Study the drawing (mm; zero at the part's minimum x, y, z) and answer. A direction names the side the tool comes from. Coordinates: 2 decimals unless noted, no trailing zeros. Order: outer loops, then holes, each group sorted by start corner. A loop starts at its lowest first (then second) coordinate and runs counter-clockwise, first axis right, second up. Notation, with made-up numbers: (43, 39) -> (71, 39) arc R12 cw to (71, 49) -> close; hole circle Ø7 at (1, 64). An arc over 180 degrees is marked (long way). Put each result on its own line as item: value. Start each with the question number.
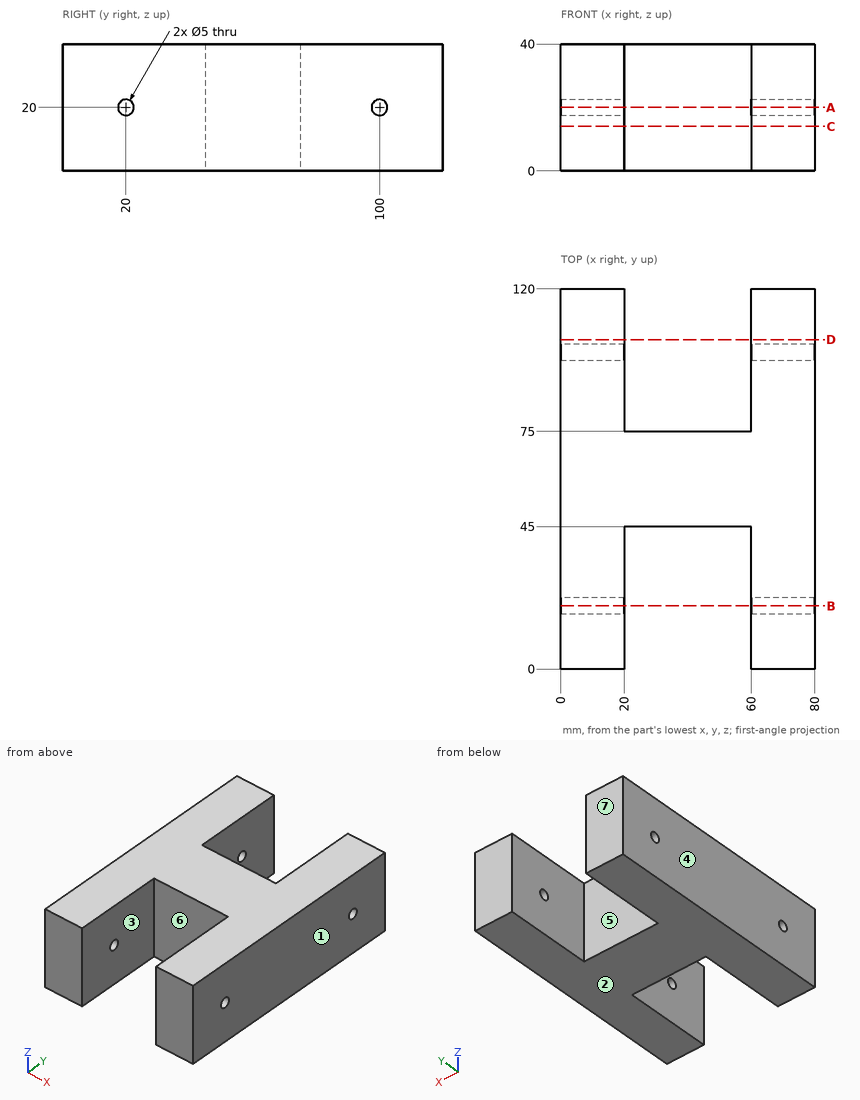
(1) For a pull along X with two mould halves and no side action, classify the marked faces 1, 2, 3 and 4 as released by +X, released by -X, zero draft, split by the parting line, or undercut.
(2) The part is cut by section C-C on z = 14. Determine the outline of the cut face in (x, y), plus the area to 3 significant figures.
(3) A tool of negligible diameter and unlimited length cuts with its end or side. For the marked faces 5, 6 and 7, from which of +Z, -Z, +X, -X, +Y, -Y can it reach the whole face along a straight path? Write none if from no direction.
(4) Find the intervals of material crossed by L1, parallel to Z at x = 70, y = 100; L2, parallel to X at y = 5, z = 8.5; L3, parallel to Y at x = 6, z = 22, in increasing order.
(5) Each of these flat-tipped pins is pushed along its axis until it touches: P1, Ø20, axis at x = 35, z = 20, coming from the +Y side; P2, Ø12, axis at x = 35.5, z = 21.5, coming from the -Y side. Where does it stop, or does it pass through?
(6) The part is cut by section B-B on y = 20. Determine the outline of the cut face in (x, z).
(7) The part is cut by section A-A on z = 20. Determine the outline of the cut face in (x, y).
(8) The part is cut by section D-D on y = 104. Determine the outline of the cut face in (x, z).
Worked out:
1. face 1: released by +X
1. face 2: zero draft
1. face 3: undercut
1. face 4: released by -X
2. outline: (0, 0) -> (20, 0) -> (20, 45) -> (60, 45) -> (60, 0) -> (80, 0) -> (80, 120) -> (60, 120) -> (60, 75) -> (20, 75) -> (20, 120) -> (0, 120) -> close
2. area: 6,000 mm2
3. face 5: +Z, -Z, +Y
3. face 6: +Z, -Z, -Y
3. face 7: +Z, -Z, +X, -X, +Y
4. L1: 0 to 17.5, 22.5 to 40
4. L2: 0 to 20, 60 to 80
4. L3: 0 to 18.5, 21.5 to 98.5, 101.5 to 120
5. P1: y = 75
5. P2: y = 45
6. outline: (0, 0) -> (20, 0) -> (20, 17.5) -> (0, 17.5) -> close; (0, 22.5) -> (20, 22.5) -> (20, 40) -> (0, 40) -> close; (60, 0) -> (80, 0) -> (80, 17.5) -> (60, 17.5) -> close; (60, 22.5) -> (80, 22.5) -> (80, 40) -> (60, 40) -> close
7. outline: (0, 0) -> (20, 0) -> (20, 17.5) -> (0, 17.5) -> close; (0, 22.5) -> (20, 22.5) -> (20, 45) -> (60, 45) -> (60, 22.5) -> (80, 22.5) -> (80, 97.5) -> (60, 97.5) -> (60, 75) -> (20, 75) -> (20, 97.5) -> (0, 97.5) -> close; (0, 102.5) -> (20, 102.5) -> (20, 120) -> (0, 120) -> close; (60, 0) -> (80, 0) -> (80, 17.5) -> (60, 17.5) -> close; (60, 102.5) -> (80, 102.5) -> (80, 120) -> (60, 120) -> close
8. outline: (0, 0) -> (20, 0) -> (20, 40) -> (0, 40) -> close; (60, 0) -> (80, 0) -> (80, 40) -> (60, 40) -> close
